For this review, take the finished solid that the model builds, in its own axes (mm). A direction names the side the tool comes from. Coordinates: 2 decimals unless noted, no trailing zeros. Write each loop counter-clockwise with the first axis right and the second up, starting at its lowest first coordinate (ties: lowest second). Pieces come first, ordered by that corner, then holes. Notation, with made-up numbers: M -40,-29 L 16,-29 A17 ccw 16,2 Z; hole C 48.5,66 d10. An arc over 180 degrees is marked long. One line per question, with ' | ' between items.
from build123d import *

# Parameters (mm, degrees)
BOSS_EXTRUDE1_DEPTH = 10
SKETCH2_R           = 4
CUT_EXTRUDE1_DEPTH  = 50.348252249
SKETCH3_R           = 1.5
CUT_EXTRUDE2_DEPTH  = 50.348252249
SKETCH5_W           = 42.5
SKETCH5_H           = 10
CUT_EXTRUDE4_DEPTH  = 2
FILLET1_R           = 10


with BuildPart() as part:
    # Sketch1 → Boss-Extrude1 (new body)
    with BuildSketch(Plane(origin=(0, 0, 0), x_dir=(1, 0, 0), z_dir=(0, 1, 0))):
        Polygon((0, 0), (0, 34), (0, 42.5), (5, 42.5), (5, 34.5), (23, 34.5), (23, 23.5), (5, 23.5), (5, -15), (0, -15), (0, -5), (-10, -5), (-10, -15), (-13, -15), (-13, 0), align=None)
    extrude(amount=BOSS_EXTRUDE1_DEPTH)

    # Sketch2 → Cut-Extrude1 (cut, through all)
    with BuildSketch(Plane(origin=(0, 10, 0), x_dir=(1, 0, 0), z_dir=(0, 1, 0))):
        with Locations((16, 25)):
            Circle(SKETCH2_R)
    extrude(amount=-CUT_EXTRUDE1_DEPTH, mode=Mode.SUBTRACT)

    # Sketch3 → Cut-Extrude2 (cut, through all)
    with BuildSketch(Plane.ZY):
        with Locations((-39.5, 7.5)):
            Circle(SKETCH3_R)
        with Locations((-20.5, 7.5)):
            Circle(SKETCH3_R)
    extrude(amount=-CUT_EXTRUDE2_DEPTH, mode=Mode.SUBTRACT)

    # Sketch5 → Cut-Extrude4 (cut)
    with BuildSketch(Plane.ZY):
        with Locations((-21.25, 5)):
            Rectangle(SKETCH5_W, SKETCH5_H)
    extrude(amount=-CUT_EXTRUDE4_DEPTH, mode=Mode.SUBTRACT)

    # Fillet1
    fillet1_edges = [part.edges().sort_by_distance(p)[0] for p in [
        (23, 5, -34.5),
    ]]
    fillet(fillet1_edges, radius=FILLET1_R)


solid = part.part
1) We need section C-C on y = 3.75. State the section outline as (x, z) points, then the cut area to 3 significant figures.
Responses:
outline: M -13,0 L 2,0 L 2,-42.5 L 5,-42.5 L 5,-34.5 L 13,-34.5 A10 ccw 23,-24.5 L 23,-23.5 L 19.71,-23.5 A4 cw long 12.29,-23.5 L 5,-23.5 L 5,15 L 0,15 L 0,5 L -10,5 L -10,15 L -13,15 Z | area: 437 mm^2
2) The part is to be moulded in two halves that separate along X. For faces 5 (the flat face through (-10, 5, 10)), 6 (the flat face through (2, 5, -22)), 7 (the cylindrical face through (3.5, 6.6, -21.7)), say which applies: +X half, -X half, draft (parallel to the pull), parting line (faces both ways), or undercut.
Responses:
face 5: undercut | face 6: -X half | face 7: draft
3) To check wall thickness, follow line 1 along X through (y, z) = (3.25, 8); line 2 along Y through (x, z) = (2.9, -20.5); line 3 along X through (y, z) = (5.75, -25). State the ranges of each line that lie inside material, in increasing order. Write a range as [from, to].
Responses:
line 1: [-13, -10], [0, 5] | line 2: [0, 6], [9, 10] | line 3: [2, 12], [20, 22.99]
4) We need section D-D on z = -7. State the section outline as (x, y) points, then the cut area to 3 significant figures.
Responses:
outline: M 2,0 L 5,0 L 5,10 L 2,10 Z | area: 30.0 mm^2
5) Machinability: for faces 1 (the flat face through (5, 5, -5)), 2 (the flat face through (-6, 5, 0)), 3 (the flat face through (-5, 5, 5)), 4 (the flat face through (9, 5, -34.5)), which of the approach directions +Z, -Z, +X, -X, +Y, -Y give a long, thin tool a straight path to every point of the face, cutting with its end or side? Answer none if there is none.
Responses:
face 1: +Z, +X, +Y, -Y | face 2: -Z, -X, +Y, -Y | face 3: +Z, +Y, -Y | face 4: -Z, +X, +Y, -Y
6) Insertion check: pin 1 Ø1.5 at (x, y) = (14.5, 8) entering from +Z; pin 2 Ø3.5 at (y, z) = (7.5, -20.5) entering from -X; pin 3 Ø4 at (y, z) = (7.5, -39.5) entering from +X. Each pin has a flat end and moves straight along its axis. Give the tip position at first contact, or say it passes through.
Responses:
pin 1: z = -28.31 | pin 2: x = 2 | pin 3: x = 5
7) We need section B-B on y = 7.5. State the section outline as (x, z) points.
Responses:
outline: M -13,0 L 2,0 L 2,-19 L 5,-19 L 5,15 L 0,15 L 0,5 L -10,5 L -10,15 L -13,15 Z; M 2,-42.5 L 5,-42.5 L 5,-41 L 2,-41 Z; M 2,-38 L 5,-38 L 5,-34.5 L 13,-34.5 A10 ccw 23,-24.5 L 23,-23.5 L 19.71,-23.5 A4 cw long 12.29,-23.5 L 5,-23.5 L 5,-22 L 2,-22 Z
8) We need section A-A on z = -39.5. State the section outline as (x, y) points.
Responses:
outline: M 2,0 L 5,0 L 5,6 L 2,6 Z; M 2,9 L 5,9 L 5,10 L 2,10 Z
